```python
from build123d import *

# Parameters (mm, degrees)
SKETCH083_W           = 85.2
SKETCH083_H           = 204
SKETCH083_W_2         = 3.2
SKETCH083_H_2         = 5.6
SKETCH083_W_3         = 7.6
PAD041_DEPTH          = 3.2
SKETCH084_R           = 2.45
PAD042_DEPTH          = 7.1
SKETCH085_W           = 1.6
SKETCH085_H           = 77.6064407756
PAD043_DEPTH          = 10.3
PAD043_DEPTH_BACK     = 14.7
POLARPATTERN003_COUNT = 2
SKETCH086_W           = 6.4
SKETCH086_H           = 3.2
PAD044_DEPTH          = 5


with BuildPart() as part:
    # Sketch083 → Pad041 (new body)
    with BuildSketch(Plane.XY.offset(-86.8064407756)):
        Rectangle(SKETCH083_W, SKETCH083_H)
        with Locations((-39.4, -72.6064407756)):
            Rectangle(SKETCH083_W_2, SKETCH083_H_2, mode=Mode.SUBTRACT)
        with Locations((-19.8, -72.6064407756)):
            Rectangle(SKETCH083_W_3, SKETCH083_H_2, mode=Mode.SUBTRACT)
        with Locations((39.4, 72.6064407756)):
            Rectangle(SKETCH083_W_2, SKETCH083_H_2, mode=Mode.SUBTRACT)
        with Locations((19.8, 72.6064407756)):
            Rectangle(SKETCH083_W_3, SKETCH083_H_2, mode=Mode.SUBTRACT)
    extrude(amount=PAD041_DEPTH)

    # Sketch084 → Pad042 (join, symmetric)
    with BuildSketch(Plane.YZ.offset(-30.7)):
        with BuildLine():
            ThreePointArc((-75.8064407756, 0), (-73.4704487226, -18.6737684351), (-66.6064407756, -36.1966643528))
            Line((-66.6064407756, -83.6064407756), (-66.6064407756, -36.1966643528))
            Line((-78.6064407756, -83.6064407756), (-66.6064407756, -83.6064407756))
            Line((-78.6064407756, 6), (-78.6064407756, -83.6064407756))
            Line((-75.8064407756, 6), (-78.6064407756, 6))
            Line((-75.8064407756, 0), (-75.8064407756, 6))
        make_face()
        with Locations((-72.6064407756, -41.4032203878)):
            Circle(SKETCH084_R, mode=Mode.SUBTRACT)
    pad042 = extrude(amount=PAD042_DEPTH, both=True)

    # Sketch085 → Pad043 (join, two sides)
    with BuildSketch(Plane.YZ.offset(-30.7)) as pad043_sk:
        with Locations((-79.4064407756, -44.8032203878)):
            Rectangle(SKETCH085_W, SKETCH085_H)
    pad043 = extrude(amount=-PAD043_DEPTH) + extrude(pad043_sk.sketch, amount=PAD043_DEPTH_BACK)

    # PolarPattern003: Pad042, Pad043 ×2 about axis
    polarpattern003_axis = Axis((0, 0, 0), (0, 0, 1))
    for i in range(1, POLARPATTERN003_COUNT):
        add(pad042.rotate(polarpattern003_axis, i * 360 / POLARPATTERN003_COUNT))
        add(pad043.rotate(polarpattern003_axis, i * 360 / POLARPATTERN003_COUNT))

    # Sketch086 → Pad044 (join)
    with BuildSketch(Plane.XY.offset(-83.6064407756)):
        Rectangle(SKETCH086_W, SKETCH086_H)
    extrude(amount=PAD044_DEPTH)


solid = part.part
```
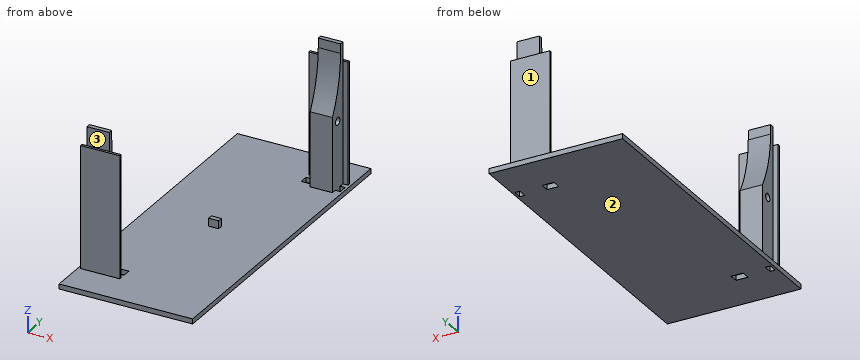
Model file for the job. Use its own axes, mm. Face numbers are marked on the shaded views. A direction names the side the tool comes from. Coordinates: 2 decimals unless noted, no trailing zeros. Loops run counter-clockwise (first coordinate to the right, second up) from the corner with the lowest first, then second, coordinate; pieces in that order, holes last. Notation, with made-up numbers: (-25, -3) -> (-8, -3) arc R18 cw to (-8, 11) -> close; hole circle Ø6 at (-7.75, 50.25). An arc over 180 degrees is marked (long way). Answer as a JSON object with one key per item and string values.
Q1. 3-axis set-ups, long thin cutter, end or side, ignore diameter. For the marked faces 1, 2 and 3: which of +Z, -Z, +X, -X, +Y, -Y reach the whole face in a straight line?
Report:
{"face 1": "+Z, +X, -X, +Y", "face 2": "-Z, +X, -X, +Y, -Y", "face 3": "+Z, +X, -X, -Y"}
Q2. Flat gauge pins, fed straight in: P1, Ø6, axis at x = -31.5, z = -1, coming from the -Y side; P2, Ø1.6, axis at x = -0.5, y = -0.5, coming from the +Z side; P3, Ø12, axis at x = -4.5, z = -23, coming from the -Y side; P4, Ø5, axis at x = 32, z = 3, coming from the -Y side. Where does each tip first touch, or does it go through?
Report:
{"P1": "stops at y = -78.61", "P2": "stops at z = -78.61", "P3": "passes through", "P4": "stops at y = 75.81"}
Q3. Cut at B-B (x = 21). List the corners of the cut face in (y, z), and give its area (3 significant figures).
Report:
{"outline": "(-102, -86.81) -> (69.81, -86.81) -> (69.81, -83.61) -> (-102, -83.61) -> close; (75.41, -86.81) -> (102, -86.81) -> (102, -83.61) -> (80.21, -83.61) -> (80.21, -6) -> (78.61, -6) -> (78.61, -83.61) -> (75.41, -83.61) -> close", "area": "759 mm2"}
Q4. Cut at D-D (x = 7). List the corners of the cut face in (y, z).
Report:
{"outline": "(-102, -86.81) -> (102, -86.81) -> (102, -83.61) -> (-102, -83.61) -> close"}
Q5. Cut at C-C (z = -23). List the corners of the cut face in (x, y).
Report:
{"outline": "(-41, -80.21) -> (-16, -80.21) -> (-16, -78.61) -> (-23.6, -78.61) -> (-23.6, -72.23) -> (-37.8, -72.23) -> (-37.8, -78.61) -> (-41, -78.61) -> close; (16, 78.61) -> (23.6, 78.61) -> (23.6, 72.23) -> (37.8, 72.23) -> (37.8, 78.61) -> (41, 78.61) -> (41, 80.21) -> (16, 80.21) -> close"}
Q6. Cut at A-A (z = -76). List the corners of the cut face in (x, y).
Report:
{"outline": "(-41, -80.21) -> (-16, -80.21) -> (-16, -78.61) -> (-23.6, -78.61) -> (-23.6, -66.61) -> (-37.8, -66.61) -> (-37.8, -78.61) -> (-41, -78.61) -> close; (16, 78.61) -> (23.6, 78.61) -> (23.6, 66.61) -> (37.8, 66.61) -> (37.8, 78.61) -> (41, 78.61) -> (41, 80.21) -> (16, 80.21) -> close"}
Q7. Probe probe 1 along X at (y, z) = (-74, -38); probe 2 along X at (y, z) = (72.5, -69); probe 3 along Z at (x, y) = (11, -74). List the from-to ranges inside material, lowest first.
Report:
{"probe 1": "x = -37.8 to -23.6", "probe 2": "x = 23.6 to 37.8", "probe 3": "z = -86.81 to -83.61"}
